```python
from build123d import *

# Parameters (mm, degrees)
CROQUIS2_W               = 118
CROQUIS2_H               = 88
SALIENTE_EXTRUIR1_DEPTH  = 5
CROQUIS3_W               = 118
CROQUIS3_H               = 88
CROQUIS3_W_2             = 112
CROQUIS3_H_2             = 82
SALIENTE_EXTRUIR2_DEPTH  = 80
CROQUIS4_W               = 150
CROQUIS4_H               = 120
SALIENTE_EXTRUIR3_DEPTH  = 5
CROQUIS7_W               = 60
CROQUIS7_H               = 17
CORTAR_EXTRUIR3_DEPTH    = 5
CROQUIS8_W               = 3
CROQUIS8_H               = 17
SALIENTE_EXTRUIR4_DEPTH  = 4
CROQUIS9_W               = 3
CROQUIS9_H               = 17
SALIENTE_EXTRUIR5_DEPTH  = 7
CROQUIS10_W              = 118
CROQUIS10_H              = 5
SALIENTE_EXTRUIR6_DEPTH  = 5
CROQUIS11_W              = 93
CROQUIS11_H              = 5
SALIENTE_EXTRUIR7_DEPTH  = 5
CROQUIS12_W              = 123
CROQUIS12_H              = 5
SALIENTE_EXTRUIR8_DEPTH  = 5
CROQUIS13_W              = 98
CROQUIS13_H              = 5
SALIENTE_EXTRUIR9_DEPTH  = 5
SALIENTE_EXTRUIR11_DEPTH = 85
CORTAR_EXTRUIR4_DEPTH    = 10
SALIENTE_EXTRUIR12_DEPTH = 70
CROQUIS21_W              = 49
CROQUIS21_H              = 17
CORTAR_EXTRUIR5_DEPTH    = 70
REDONDEO4_R              = 10
REDONDEO5_R              = 100
SALIENTE_EXTRUIR13_DEPTH = 20
CROQUIS23_W              = 143.80914693
CROQUIS23_H              = 144.72077086
CROQUIS23_R              = 24.004265162
SALIENTE_EXTRUIR14_DEPTH = 5
SALIENTE_EXTRUIR15_DEPTH = 5
REDONDEO9_R              = 20
CROQUIS27_W              = 105.325741151
CROQUIS27_H              = 5
CORTAR_EXTRUIR7_DEPTH    = 210.21942266
CROQUIS28_W              = 104.72077086
CROQUIS28_H              = 5
CORTAR_EXTRUIR8_DEPTH    = 143.809145
CROQUIS29_R              = 2.5
CORTAR_EXTRUIR9_DEPTH    = 10
REDONDEO10_R             = 20
CROQUIS30_W              = 82
CROQUIS30_H              = 69.590652645
CORTAR_EXTRUIR10_DEPTH   = 30


with BuildPart() as part:
    # Croquis2 → Saliente-Extruir1 (new body)
    with BuildSketch(Plane(origin=(0, 0, 0), x_dir=(1, 0, 0), z_dir=(0, 1, 0))):
        Rectangle(CROQUIS2_W, CROQUIS2_H)
    extrude(amount=SALIENTE_EXTRUIR1_DEPTH)

    # Croquis3 → Saliente-Extruir2 (add)
    with BuildSketch(Plane(origin=(0, 5, 0), x_dir=(1, 0, 0), z_dir=(0, 1, 0))):
        Rectangle(CROQUIS3_W, CROQUIS3_H)
        Rectangle(CROQUIS3_W_2, CROQUIS3_H_2, mode=Mode.SUBTRACT)
    extrude(amount=SALIENTE_EXTRUIR2_DEPTH)

    # Croquis4 → Saliente-Extruir3 (add)
    with BuildSketch(Plane.XZ):
        Rectangle(CROQUIS4_W, CROQUIS4_H)
    extrude(amount=-SALIENTE_EXTRUIR3_DEPTH)

    # Croquis7 → Cortar-Extruir3 (cut)
    with BuildSketch(Plane.ZY.offset(59)):
        with Locations((-3, 21.5)):
            Rectangle(CROQUIS7_W, CROQUIS7_H)
    extrude(amount=-CORTAR_EXTRUIR3_DEPTH, mode=Mode.SUBTRACT)

    # Croquis8 → Saliente-Extruir4 (add)
    with BuildSketch(Plane.XY.offset(-33)):
        with Locations((-57.5, 21.5)):
            Rectangle(CROQUIS8_W, CROQUIS8_H)
    extrude(amount=SALIENTE_EXTRUIR4_DEPTH)

    # Croquis9 → Saliente-Extruir5 (add)
    with BuildSketch(Plane(origin=(0, 0, 27), x_dir=(-1, 0, 0), z_dir=(0, 0, -1))):
        with Locations((57.5, 21.5)):
            Rectangle(CROQUIS9_W, CROQUIS9_H)
    extrude(amount=SALIENTE_EXTRUIR5_DEPTH)

    # Croquis10 → Saliente-Extruir6 (add)
    with BuildSketch(Plane.XY.offset(44)):
        with Locations((0, 72.5)):
            Rectangle(CROQUIS10_W, CROQUIS10_H)
    extrude(amount=SALIENTE_EXTRUIR6_DEPTH)

    # Croquis11 → Saliente-Extruir7 (add)
    with BuildSketch(Plane(origin=(59, 0, 0), x_dir=(0, 0, -1), z_dir=(1, 0, 0))):
        with Locations((-2.5, 72.5)):
            Rectangle(CROQUIS11_W, CROQUIS11_H)
    extrude(amount=SALIENTE_EXTRUIR7_DEPTH)

    # Croquis12 → Saliente-Extruir8 (add)
    with BuildSketch(Plane(origin=(0, 0, -44), x_dir=(-1, 0, 0), z_dir=(0, 0, -1))):
        with Locations((-2.5, 72.5)):
            Rectangle(CROQUIS12_W, CROQUIS12_H)
    extrude(amount=SALIENTE_EXTRUIR8_DEPTH)

    # Croquis13 → Saliente-Extruir9 (add)
    with BuildSketch(Plane.ZY.offset(59)):
        with Locations((0, 72.5)):
            Rectangle(CROQUIS13_W, CROQUIS13_H)
    extrude(amount=SALIENTE_EXTRUIR9_DEPTH)

    # Croquis16 → Saliente-Extruir11 (add)
    with BuildSketch(Plane(origin=(0, 0, 0), x_dir=(-1, 0, 0), z_dir=(0, -1, 0))):
        with BuildLine():
            Line((-59, 44), (16.214965512, 44))
            ThreePointArc((16.214965512, 44), (-105.589495195, 0), (16.214965512, -44))
            Line((16.214965512, -44), (-59, -44))
            Line((-59, -44), (-59, 44))
        make_face()
    extrude(amount=-SALIENTE_EXTRUIR11_DEPTH)

    # Croquis18 → Cortar-Extruir4 (cut)
    with BuildSketch(Plane(origin=(0, 85, 0), x_dir=(1, 0, 0), z_dir=(0, 1, 0))):
        Polygon((-64, 49), (-8.415102712, 49), (63.361111922, 49), (64, 49), (64, 44), (64, -44), (64, -49), (63.361111922, -49), (-8.415102712, -49), (-64, -49), (-64, -44), (-16.214965512, -44), (59, -44), (59, 44), (-16.214965512, 44), (-64, 44), align=None)
    extrude(amount=-CORTAR_EXTRUIR4_DEPTH, mode=Mode.SUBTRACT)

    # Croquis19 → Saliente-Extruir12 (add)
    with BuildSketch(Plane(origin=(0, 5, 0), x_dir=(1, 0, 0), z_dir=(0, 1, 0))):
        Polygon((-16.214965512, -44), (-59, -44), (-59, 44), (-16.214965512, 44), (3.50341587, 44), (3.50341587, 49), (-8.415102712, 49), (-64, 49), (-64, -49), (-8.415102712, -49), (4.243498443, -49), (4.243498443, -44), align=None)
    extrude(amount=SALIENTE_EXTRUIR12_DEPTH)

    # Croquis21 → Cortar-Extruir5 (cut)
    with BuildSketch(Plane(origin=(-56, 0, 0), x_dir=(0, 0, -1), z_dir=(1, 0, 0))):
        with Locations((4.5, 21.5)):
            Rectangle(CROQUIS21_W, CROQUIS21_H)
    extrude(amount=-CORTAR_EXTRUIR5_DEPTH, mode=Mode.SUBTRACT)

    # Redondeo4
    redondeo4_edges = [part.edges().sort_by_distance(p)[0] for p in [
        (-64, 40, -49),
        (-64, 40, 49),
    ]]
    fillet(redondeo4_edges, radius=REDONDEO4_R)

    # Redondeo5
    redondeo5_edges = [part.edges().sort_by_distance(p)[0] for p in [
        (-11.625579702, 40, -49),
        (-11.625579702, 40, 49),
    ]]
    fillet(redondeo5_edges, radius=REDONDEO5_R)

    # Croquis22 → Saliente-Extruir13 (add)
    with BuildSketch(Plane(origin=(0, 85, 0), x_dir=(1, 0, 0), z_dir=(0, 1, 0))):
        with BuildLine():
            Line((64, -49), (4.315842741, -49))
            Line((4.315842741, -49), (-11.625579493, -49))
            ThreePointArc((-11.625579493, -49), (105.589495048, 0), (-11.625579493, 49))
            Line((-11.625579493, 49), (4.315842741, 49))
            Line((4.315842741, 49), (64, 49))
            Line((64, 49), (64, -49))
        make_face()
    extrude(amount=SALIENTE_EXTRUIR13_DEPTH)

    # Croquis23 → Saliente-Extruir14 (add)
    with BuildSketch(Plane(origin=(0, 0, 0), x_dir=(-1, 0, 0), z_dir=(0, -1, 0))):
        with Locations((-36.740101048, 0)):
            Rectangle(CROQUIS23_W, CROQUIS23_H)
        with Locations((-36.740101048, 0)):
            Circle(CROQUIS23_R, mode=Mode.SUBTRACT)
    extrude(amount=-SALIENTE_EXTRUIR14_DEPTH)

    # Croquis25 → Saliente-Extruir15 (add)
    with BuildSketch(Plane(origin=(0, 0, 0), x_dir=(-1, 0, 0), z_dir=(0, -1, 0))):
        Polygon((35.164472417, -60), (35.164472417, -72.36038543), (-108.644674513, -72.36038543), (-108.644674513, 72.36038543), (35.164472417, 72.36038543), (35.164472417, 60), (75, 60), (75, -60), align=None)
    extrude(amount=SALIENTE_EXTRUIR15_DEPTH)

    # Redondeo9
    # the kernel refuses this fillet: 20 mm, written as the material it takes off along each edge
    with BuildSketch(Plane(origin=(108.644674513, -55, -72.36038543), x_dir=(-1, 0, 0), z_dir=(0, 1, 0)), Plane(origin=(108.644674513, -55, 72.36038543), x_dir=(0, 0, -1), z_dir=(0, 1, 0))) as redondeo9_piece_1:
        with BuildLine():
            CenterArc((REDONDEO9_R, REDONDEO9_R), REDONDEO9_R, 180, 90)
            Line((0, REDONDEO9_R), (-REDONDEO9_R * 0.02, REDONDEO9_R))
            Line((-REDONDEO9_R * 0.02, REDONDEO9_R), (-REDONDEO9_R * 0.02, -REDONDEO9_R * 0.02))
            Line((-REDONDEO9_R * 0.02, -REDONDEO9_R * 0.02), (REDONDEO9_R, -REDONDEO9_R * 0.02))
            Line((REDONDEO9_R, -REDONDEO9_R * 0.02), (REDONDEO9_R, 0))
        make_face()
    extrude(amount=110, mode=Mode.SUBTRACT)
    with BuildSketch(Plane(origin=(-35.164472417, -51.20851445, 72.36038543), x_dir=(1, 0, 0), z_dir=(0, 1, 0))) as redondeo9_piece_2:
        with BuildLine():
            CenterArc((18.48340578, 20), REDONDEO9_R, 202.456427621, 67.543572379)
            Line((0, 12.36038543), (-0.369668116, 12.207593139))
            ThreePointArc((-0.369668116, 12.207593139), (-0.4, 6.180192715), (-0.4, 0))
            Line((-0.4, 0), (0, -0.4))
            Line((0, -0.4), (18.48340578, -0.4))
            Line((18.48340578, -0.4), (18.48340578, 0))
        make_face()
    extrude(amount=102.417028899, mode=Mode.SUBTRACT)
    with BuildSketch(Plane(origin=(-35.164472417, -51.20851445, -72.36038543), x_dir=(0, 0, 1), z_dir=(0, 1, 0))) as redondeo9_piece_3:
        with BuildLine():
            CenterArc((20, 18.48340578), REDONDEO9_R, 180, 67.543572379)
            Line((0, 18.48340578), (-0.4, 18.48340578))
            Line((-0.4, 18.48340578), (-0.4, 0))
            Line((-0.4, 0), (0, -0.4))
            ThreePointArc((0, -0.4), (6.180192715, -0.4), (12.207593139, -0.369668116))
            Line((12.207593139, -0.369668116), (12.36038543, 0))
        make_face()
    extrude(amount=102.417028899, mode=Mode.SUBTRACT)

    # Croquis27 → Cortar-Extruir7 (cut, through all)
    with BuildSketch(Plane(origin=(0, 0, -72.36038543), x_dir=(-1, 0, 0), z_dir=(0, 0, -1))):
        with Locations((-35.981803938, -2.5)):
            Rectangle(CROQUIS27_W, CROQUIS27_H)
    extrude(amount=-CORTAR_EXTRUIR7_DEPTH, mode=Mode.SUBTRACT)

    # Croquis28 → Cortar-Extruir8 (cut)
    with BuildSketch(Plane(origin=(108.644674513, 0, 0), x_dir=(0, 0, -1), z_dir=(1, 0, 0))):
        with Locations((0, -2.5)):
            Rectangle(CROQUIS28_W, CROQUIS28_H)
    extrude(amount=-CORTAR_EXTRUIR8_DEPTH, mode=Mode.SUBTRACT)

    # Croquis29 → Cortar-Extruir9 (cut)
    with BuildSketch(Plane(origin=(0, -5, 0), x_dir=(-1, 0, 0), z_dir=(0, -1, 0))):
        with Locations(Location((-96.256800969, -61.48231173, 0), (0, 0, 90))):
            Circle(CROQUIS29_R)
        with Locations(Location((-97.464115668, 60.274997031, 0), (0, 0, 90))):
            Circle(CROQUIS29_R)
        with Locations(Location((24.293193094, 61.48231173, 0), (0, 0, 90))):
            Circle(CROQUIS29_R)
        with Locations(Location((25.500507793, -60.274997031, 0), (0, 0, 90))):
            Circle(CROQUIS29_R)
    extrude(amount=-CORTAR_EXTRUIR9_DEPTH, mode=Mode.SUBTRACT)

    # Redondeo10
    redondeo10_edges = [part.edges().sort_by_distance(p)[0] for p in [
        (-75, 0, -60),
        (-75, 0, 60),
    ]]
    fillet(redondeo10_edges, radius=REDONDEO10_R)

    # Croquis30 → Cortar-Extruir10 (cut)
    with BuildSketch(Plane.ZY.offset(-56)):
        with Locations((0, 39.795326323)):
            Rectangle(CROQUIS30_W, CROQUIS30_H)
    extrude(amount=-CORTAR_EXTRUIR10_DEPTH, mode=Mode.SUBTRACT)


solid = part.part
```
Source: CAD feature listing. Evaluate the final solid. Frame: model axes, mm. A direction names the side the tool comes from. Round coordinates to 2 decimals unless told otherwise and drop trailing zeros. Write each loop counter-clockwise with the first axis right and the second up, starting at its lowest first coordinate (ties: lowest second). Pieces come first, ordered by that corner, then holes. Notation, with made-up numbers: M 13.25,49.25 L 49.25,49.25 A10 cw 49.25,56.25 Z; hole C 2.25,41 d2. An arc over 180 degrees is marked long. Answer as a JSON object with one key per item and string values. Group by question number.
(1) Section query B-B on z = 0. Output: boundary loops of the cut face in (x, y), then the cut area to 3 significant figures.
(2) Section query A-A on y = 80.5. Output: boundary loops of the cut face in (x, z).
(3) Ray query, line 1 (Y direction, x = 68, z = 10); line 2 (Y direction, x = 19.5, z = 61); line 3 (Y direction, x = -46, z = 24). Return the intervals inside material, ascending. Write a range as [from, to].
(4) First-contact query: pin 1 (5 mm diameter, centred on x = 47, y = 78.5, fed in from +Z); pin 2 (6 mm diameter, centred on x = 3, y = 13.5, fed in from +Z); pin 3 (1 mm diameter, centred on x = 81.5, z = 6.5, fed in from -Y); pin 4 (6.5 mm diameter, centred on x = 97.46, z = -60.27, fed in from -Y). Flat tips, straight axial feed; report the tip coordinate or a pass-through.
(5) Mould query, pull axis Y, two halves, no side actions, for faces 1 (the flat face through (71, 74.591, -1)), 2 (the flat face through (99, -5, 60)), 3 (the flat face through (-64, 40, -1)). Classes: +Y half, -Y half, draft (parallel to the pull), parting line (faces both ways), or undercut.
(6) Section query C-C on x = -49.5. Output: boundary loops of the cut face in (y, z).
(7) Reachability of faces 4 (the flat face through (-59, 80, 1)), 5 (the flat face through (-60, 30, -5)), 6 (the flat face through (88.645, -3, 62)), 7 (the flat face through (27, 90, 49)) from +Z, -Z, +X, -X, +Y, -Y: full face, straight path, thin tool, end or side. Return the list, or none.
(8) Section query D-D on y = 35. Output: boundary loops of the cut face in (x, z), then the cut area to 3 significant figures.
Computed values:
{
 "1": {"outline": "M -75,-5 L -35.16,-5 L -35.16,0 L 108.64,0 L 108.64,5 L 105.59,5 L 105.59,105 L 64,105 L 64,75 L 59,75 L 59,85 L 56,85 L 56,74.59 L 86,74.59 L 86,5 L -56,5 L -56,13 L -64,13 L -64,5 L -75,5 Z; M -64,30 L -56,30 L -56,85 L -59,85 L -59,75 L -64,75 Z", "area": "4,230 mm^2"},
 "2": {"outline": "M -59,-44 L 59,-44 L 59,44 L -59,44 Z; M -11.63,-49 A68.85 ccw long -11.63,49 L 64,49 L 64,-49 Z; hole M -56,-41 L 56,-41 L 56,41 L -56,41 Z"},
 "3": {"line 1": "[0, 5], [74.59, 105]", "line 2": "[0, 105]", "line 3": "[-5, 5]"},
 "4": {"pin 1": "z = 68.41", "pin 2": "z = 61.61", "pin 3": "y = 0", "pin 4": "y = -5"},
 "5": {"face 1": "undercut", "face 2": "-Y half", "face 3": "draft"},
 "6": {"outline": "M -5,-60 L 5,-60 L 5,-49 L 75,-49 L 75,-44 L 85,-44 L 85,-41 L 5,-41 L 5,41 L 85,41 L 85,44 L 75,44 L 75,49 L 5,49 L 5,60 L -5,60 Z"},
 "7": {"face 4": "+Z, -Z, -X, +Y", "face 5": "-X", "face 6": "+Z, -Z, -Y", "face 7": "-X, +Y"},
 "8": {"outline": "M -64,-39 A10 ccw -54,-49 L -42.69,-49 A100 cw 4.35,-60.76 A68.85 ccw long 4.35,60.76 A100 cw -42.69,49 L -54,49 A10 ccw -64,39 Z; hole M -56,-41 L 86,-41 L 86,41 L -56,41 Z", "area": "7,110 mm^2"}
}
